from build123d import *

# Parameters (mm, degrees)
BOSS_EXTRUDE1_DEPTH      = 12.5
BOSS_EXTRUDE1_DEPTH_BACK = 12.5
SKETCH11_R               = 7.5
BOSS_EXTRUDE4_DEPTH      = 180
BOSS_EXTRUDE4_DEPTH_BACK = 180
SKETCH12_W               = 25
SKETCH12_H               = 70
BOSS_EXTRUDE5_DEPTH      = 40
SKETCH13_W               = 20
SKETCH13_H               = 40
CUT_EXTRUDE2_DEPTH       = 70
SKETCH15_R               = 2.5
CUT_EXTRUDE3_DEPTH       = 191
CUT_EXTRUDE3_DEPTH_BACK  = 171
BOSS_EXTRUDE8_DEPTH      = 20


with BuildPart() as part:
    # Sketch1 → Boss-Extrude1 (new body, two sides)
    with BuildSketch(Plane(origin=(0, 0, 0), x_dir=(0, 0, -1), z_dir=(1, 0, 0))) as boss_extrude1_sk:
        with BuildLine():
            Line((10, 28.284271247), (10, 264.811253537))
            ThreePointArc((10, 264.811253537), (-46.581095136, 260.873918926), (-101.028366233, 244.986263322))
            Line((-101.028366233, 244.986263322), (-161.650144498, 209.986263322))
            Line((-161.650144498, 209.986263322), (-152.500136319, 198.100248417))
            ThreePointArc((-152.500136319, 198.100248417), (-85.263049352, 235.011089984), (-10, 249.799919936))
            Line((-10, 249.799919936), (-10, 28.284271247))
            ThreePointArc((-10, 28.284271247), (0, -30), (10, 28.284271247))
        make_face()
    extrude(amount=BOSS_EXTRUDE1_DEPTH)
    extrude(boss_extrude1_sk.sketch, amount=-BOSS_EXTRUDE1_DEPTH_BACK)

    # Sketch11 → Boss-Extrude4 (add, two sides)
    with BuildSketch(Plane(origin=(0, 0, 0), x_dir=(0, 0, -1), z_dir=(1, 0, 0))) as boss_extrude4_sk:
        Circle(SKETCH11_R)
    extrude(amount=BOSS_EXTRUDE4_DEPTH)
    extrude(boss_extrude4_sk.sketch, amount=-BOSS_EXTRUDE4_DEPTH_BACK)

    # Sketch12 → Boss-Extrude5 (add)
    with BuildSketch(Plane(origin=(0, 227.486263322, 131.339255366), x_dir=(1, 0, 0), z_dir=(0, 0.866025404, 0.5))):
        Rectangle(SKETCH12_W, SKETCH12_H)
    extrude(amount=BOSS_EXTRUDE5_DEPTH)

    # Sketch13 → Cut-Extrude2 (cut)
    with BuildSketch(Plane(origin=(0, 17.5, -30.310889132), x_dir=(-1, 0, 0), z_dir=(0, 0.5, -0.866025404))):
        with Locations((0, 282.678510731)):
            Rectangle(SKETCH13_W, SKETCH13_H)
    extrude(amount=-CUT_EXTRUDE2_DEPTH, mode=Mode.SUBTRACT)

    # Sketch15 → Cut-Extrude3 (cut, two sides)
    with BuildSketch(Plane.ZY.offset(-10)) as cut_extrude3_sk:
        with Locations((146.114255366, 253.077314003)):
            Circle(SKETCH15_R)
    extrude(amount=CUT_EXTRUDE3_DEPTH, mode=Mode.SUBTRACT)
    extrude(cut_extrude3_sk.sketch, amount=-CUT_EXTRUDE3_DEPTH_BACK, mode=Mode.SUBTRACT)

    # Sketch16 → Boss-Extrude8 (add)
    with BuildSketch(Plane.ZY.offset(-10)):
        Polygon((122.098874309, 241.48145385), (124.598874309, 245.811580869), (150.579636422, 230.811580869), (148.079636422, 226.48145385), align=None)
    extrude(amount=BOSS_EXTRUDE8_DEPTH)


solid = part.part
Geometry check sheet. Reference: the model listing, model coordinates, mm. A direction names the side the tool comes from. Round coordinates to 2 decimals unless told otherwise and drop trailing zeros. Order: outer loops, then holes, each group sorted by start corner. A loop starts at its lowest first (then second) coordinate and runs counter-clockwise, first axis right, second up. Notation, with made-up numbers: (9.5, 83) - (27.5, 83) arc R26 ccw to (27.5, 115) - close; hole circle Ø11 at (2, 73). An arc over 180 degrees is marked (long way). One line per question, with ' | ' between items. Start each with the question number.
(1) Sectioned sample at C-C on x = 20.5. Record the cut outline in (y, z), and give its area (3 significant figures).
(2) Access from +Z, -Z, +X, -X, +Y, -Y to the whole of each face (thin tool, end or side, straight path). Record for faces 4 (the flat face through (0.14, 233.876, 135.271)), 5 (the cylindrical face through (-95.078, 0.33, 7.493)), 6 (the flat face through (0, 145, -10)), 7 (the cylindrical face through (0.175, 261.013, 45.798)), 8 (the flat face through (0.14, 238.417, 137.407)).
(3) Depth check by flat-ended pin: pin 1 Ø4 at (y, z) = (253.08, 146.11) entering from -X; pin 2 Ø7.5 at (x, y) = (2.5, 139) entering from +Z. Enter the tip coordinate at first touch or a pass-through.
(4) Sectioned sample at A-A on z = 0. Record the cut outline in (x, y), and give its area (3 significant figures).
(5) Release check for a two-part mould opening along Z. For faces 1 (the flat face through (-11.268, 262.064, 110.888)), 2 (the flat face through (11.232, 262.372, 150.915)), 3 (the cylindrical face through (0.175, -29.977, 1.176)) record: released by +Z, released by -Z, zero draft, split by the parting line, or undercut.
(6) Thickness scan on L1, parallel to Z at x = -8.5, y = 169; L2, parallel to Y at x = 2, z = 17.5; L3, parallel to Y at x = -7.5, z = 68. Record the ranges inside material, lowest first. Write a range as [from, to].
(7) Sectioned sample at B-B on y = 0. Record the cut outline in (x, z), and give its area (4 significant figures).
(8) Sectioned sample at D-D on y = 68. Record the cut outline in (x, z), and give its area (3 significant figures).
Conclusion:
1) outline: circle Ø15 at (0, 0) | area: 177 mm2
2) face 4: none | face 5: -X | face 6: -Z, +X, -X, +Y | face 7: +X, -X, +Y | face 8: +Z, +Y
3) pin 1: passes through | pin 2: stops at z = 10
4) outline: (-180, -7.5) - (-12.5, -7.5) - (-12.5, -30) - (12.5, -30) - (12.5, -7.5) - (180, -7.5) - (180, 7.5) - (12.5, 7.5) - (12.5, 265) - (-12.5, 265) - (-12.5, 7.5) - (-180, 7.5) - close | area: 12,400 mm2
5) face 1: undercut | face 2: released by +Z | face 3: split by the parting line
6) L1: z = [-10, 10] | L2: y = [-24.37, 24.37], [249.39, 264.42] | L3: y = [240.57, 256.13]
7) outline: (-180, -7.5) - (-12.5, -7.5) - (-12.5, -30) - (12.5, -30) - (12.5, -7.5) - (180, -7.5) - (180, 7.5) - (12.5, 7.5) - (12.5, 30) - (-12.5, 30) - (-12.5, 7.5) - (-180, 7.5) - close | area: 6,525 mm2
8) outline: (-12.5, -10) - (12.5, -10) - (12.5, 10) - (-12.5, 10) - close | area: 500 mm2
